Input: part model. Units: mm. Frame: model coordinates. Coordinates: 2 decimals unless noted, no trailing zeros. Write each loop counter-clockwise with the first axis right and the second up, starting at its lowest first coordinate (ties: lowest second). Pieces come first, ordered by that corner, then holes. Notation, with made-up numbers: (-16.5, 5) - (10.5, 5) arc R21 ccw to (10.5, 20) - close; hole circle Ø3 at (-25.5, 76). An arc over 180 degrees is marked (long way). One line per question, with ' | ' between items. Start each with the question number.
1) Line query: line 1 (Z direction, x = 0.65, y = 0.5); line 2 (Y direction, x = 0.3, z = 0.25). Output: solid intervals per line, ascending.
2) First-contact query: P1, Ø1, axis at x = 1, y = 2.5, coming from the +Z side; P2, Ø1, axis at x = 0.5, z = -2, coming from the -Y side; P3, Ø1, axis at x = 1, z = -2, coming from the +Y side. Flat tips, straight axial feed; report the tip coordinate or a pass-through.
3) Section query B-B on z = -3. Return loops of the section in (x, y), and give its area (3 significant figures).
4) Section query A-A on x = 0.9. Return loops of the section in (y, z).
5) Section query C-C on z = 2.75. Return loops of the section in (x, y).
6) Draft query along Y for faces 1 (the flat face through (0.89, -1.92, -1.97)), 2 (the cylindrical face through (0.91, -0.03, -0.61)), 3 (the flat face through (1.8, -1, 1)). Return one class per face: released by +Y, released by -Y, zero draft, split by the parting line, or undercut.
Autodesk Inventor part; units mm, degrees
ref_plane "Work Plane1" through (11.1463, 0, 0) normal (0, 0.7071, -0.7071) x (-1, 0, 0)
ref_plane "YZ Plane" through (0, 0, 0) normal (1, 0, 0) x (0, 1, 0)
ref_plane "XZ Plane" through (0, 0, 0) normal (0, 1, 0) x (-1, 0, 0)
sketch "Sketch1" plane through (0, 0, 0) normal (1, 0, 0) x (0, 1, 0)
  line L0 (0, -3.8891) -> (-3.8891, 0)
  line L1 (-3.8891, 0) -> (0, 3.8891)
  line L2 (0, 3.8891) -> (3.8891, 0)
  line L3 (3.8891, 0) -> (0, -3.8891)
  line L4 (-3.1678, 0) -> (3.1678, 0)
  point P0 (0, 0)
  point P1 (0, 0)
  dimension "d0" = 7.7782
extrude "Body" add sketch "Sketch1" along normal blind 1.8
sketch "Sketch2" plane through (0, 0, 0) normal (-1, 0, 0) x (0, 0, 1)
  point P0 (0, 0)
  point P1 (0, 0)
hole "Thread" at (0, 0, 0) direction (1, 0, 0) diameter 1.221 end through all
chamfer "Chamfer1" distance 0.2706 angle 30 1 edges at (0, 0, -0.6105) measured on face at (0, -1.4313, 1.4487)
chamfer "Chamfer2" distance 0.2706 angle 30 1 edges at (1.8, 0, -0.6105) measured on face at (1.8, -1.4313, 1.4487)
ref_plane "Work Plane1" through (11.1463, 0, 0) normal (0, 0.7071, -0.7071) x (-1, 0, 0)
equation "\"d0\" = 1.41421 * SW"
equation "\"d1\" = KOH"
equation "\"d3\" = -0.5 * GD1 + 0.5 * NND"
equation "\"d35\" = -0.5 * GD1 + 0.5 * NND"
equation "\"d5\" = -0.5 * GD1 + 0.5 * NND"
equation "\"d36\" = -0.5 * GD1 + 0.5 * NND"
equation "\"NND\" = 3"
equation "\"KOH\" = 1.8"
equation "\"SW\" = 5.5"
equation "\"GUL\" = 0.541266 * PTC"
equation "\"THREADDIA\" = 3"
equation "\"TOA\" = 30deg"
equation "\"PTC\" = 0.5"
equation "\"E0\" = 7"
equation "\"GAL\" = 0.541266 * PTC"
properties part number "DIN 562 - M3" material "Steel, Mild"
Answer key:
1) line 1: -3.39 to -0.35, 0.35 to 3.39 | line 2: -3.64 to -0.56, 0.56 to 3.64
2) P1: z = 1.89 | P2: y = -2.39 | P3: y = 2.39
3) outline: (0, -0.89) - (1.8, -0.89) - (1.8, 0.89) - (0, 0.89) - close | area: 3.20 mm²
4) outline: (-3.89, 0) - (0, -3.89) - (3.89, 0) - (0, 3.89) - close; hole circle Ø1.22 at (0, 0)
5) outline: (0, -1.14) - (1.8, -1.14) - (1.8, 1.14) - (0, 1.14) - close
6) face 1: released by -Y | face 2: undercut | face 3: zero draft
